Part model, mm, in its own coordinate system. Give positions to 0.01 mm unless a question says otherwise; leave off trailing zeros. Write each loop counter-clockwise with the first axis right and the second up, starting at its lowest first coordinate (ties: lowest second). Pieces come first, ordered by that corner, then holes. Notation, with made-up numbers: M -19,-13 L 21,-13 A16 ccw 21,15 Z; hole C 38.5,-29 d1. An arc over 180 degrees is marked long. Answer as CSV lines item,"result". Start each with the question number.
1) Slice it at B-B, the plane y = 65. Give the cut face in (x, z).
2) Slice it at D-D, the plane y = -54. Give the cut face in (x, z).
3) Wall check: line 1 along Y through (x, z) = (0, 1.3); line 2 along X through (y, z) = (-13, 22); line 3 along Y through (x, z) = (-40.5, 14.5). Give the ranges that are in metal, low to high. Write a range as from..to.
4) Pin check, flat tips, straight feed: pin 1 Ø1.5 at (x, y) = (9.5, -29.5) entering from -Z; pin 2 Ø10 at (y, z) = (41.5, 10.5) entering from -X; pin 3 Ø1.6 at (y, z) = (68, 1.5) entering from +X; pin 4 Ø1.6 at (y, z) = (63.5, 1.5) entering from -X. Stop position of each tip, or through.
5) Slice it at A-A, the plane x = 0. Give the cut face in (y, z).
6) Slice it at C-C, the plane z = 19.5. Give the cut face in (x, y).
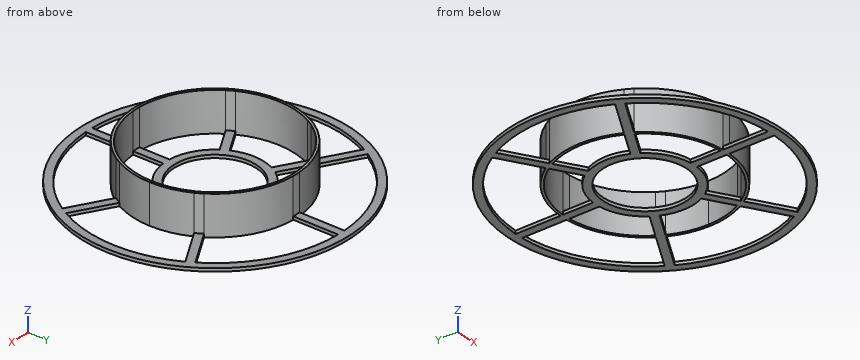
```python
from build123d import *

# Parameters (mm, degrees)
F0_R     = 85
F0_R_2   = 26
F1_DEPTH = 2
F2_DEPTH = 25


with BuildPart() as f1:
    # F0 (on Top) → F1 (new body)
    with BuildSketch(Plane.XY):
        Circle(F0_R)
        with BuildLine():
            ThreePointArc((43.384432, 27.934765), (44.686911, 25.8), (45.884432, 23.604638))
            Line((45.884432, 23.604638), (70.498195, 37.8154))
            ThreePointArc((70.498195, 37.8154), (80, 0), (70.498195, -37.8154))
            Line((70.498195, -37.8154), (45.884432, -23.604638))
            ThreePointArc((45.884432, -23.604638), (44.686911, -25.8), (43.384432, -27.934765))
            Line((43.384432, -27.934765), (67.998195, -42.145527))
            ThreePointArc((67.998195, -42.145527), (40, -69.282032), (2.5, -79.960928))
            Line((2.5, -79.960928), (2.5, -51.539402))
            ThreePointArc((2.5, -51.539402), (0, -51.6), (-2.5, -51.539402))
            Line((-2.5, -51.539402), (-2.5, -79.960928))
            ThreePointArc((-2.5, -79.960928), (-40, -69.282032), (-67.998195, -42.145527))
            Line((-67.998195, -42.145527), (-43.384432, -27.934765))
            ThreePointArc((-43.384432, -27.934765), (-44.686911, -25.8), (-45.884432, -23.604638))
            Line((-45.884432, -23.604638), (-70.498195, -37.8154))
            ThreePointArc((-70.498195, -37.8154), (-80, 0), (-70.498195, 37.8154))
            Line((-70.498195, 37.8154), (-45.884432, 23.604638))
            ThreePointArc((-45.884432, 23.604638), (-44.686911, 25.8), (-43.384432, 27.934765))
            Line((-43.384432, 27.934765), (-67.998195, 42.145527))
            ThreePointArc((-67.998195, 42.145527), (-40, 69.282032), (-2.5, 79.960928))
            Line((-2.5, 79.960928), (-2.5, 51.539402))
            ThreePointArc((-2.5, 51.539402), (0, 51.6), (2.5, 51.539402))
            Line((2.5, 51.539402), (2.5, 79.960928))
            ThreePointArc((2.5, 79.960928), (40, 69.282032), (67.998195, 42.145527))
            Line((67.998195, 42.145527), (43.384432, 27.934765))
        make_face(mode=Mode.SUBTRACT)
        with BuildLine():
            Line((28.009344, 13.284451), (44.49711, 22.803667))
            ThreePointArc((44.49711, 22.803667), (43.30127, 25), (41.99711, 27.133794))
            Line((41.99711, 27.133794), (25.509344, 17.614578))
            ThreePointArc((25.509344, 17.614578), (15.5, 26.846788), (2.5, 30.899029))
            Line((2.5, 30.899029), (2.5, 49.937461))
            ThreePointArc((2.5, 49.937461), (0, 50), (-2.5, 49.937461))
            Line((-2.5, 49.937461), (-2.5, 30.899029))
            ThreePointArc((-2.5, 30.899029), (-15.5, 26.846788), (-25.509344, 17.614578))
            Line((-25.509344, 17.614578), (-41.99711, 27.133794))
            ThreePointArc((-41.99711, 27.133794), (-43.30127, 25), (-44.49711, 22.803667))
            Line((-44.49711, 22.803667), (-28.009344, 13.284451))
            ThreePointArc((-28.009344, 13.284451), (-31, 0), (-28.009344, -13.284451))
            Line((-28.009344, -13.284451), (-44.49711, -22.803667))
            ThreePointArc((-44.49711, -22.803667), (-43.30127, -25), (-41.99711, -27.133794))
            Line((-41.99711, -27.133794), (-25.509344, -17.614578))
            ThreePointArc((-25.509344, -17.614578), (-15.5, -26.846788), (-2.5, -30.899029))
            Line((-2.5, -30.899029), (-2.5, -49.937461))
            ThreePointArc((-2.5, -49.937461), (0, -50), (2.5, -49.937461))
            Line((2.5, -49.937461), (2.5, -30.899029))
            ThreePointArc((2.5, -30.899029), (15.5, -26.846788), (25.509344, -17.614578))
            Line((25.509344, -17.614578), (41.99711, -27.133794))
            ThreePointArc((41.99711, -27.133794), (43.30127, -25), (44.49711, -22.803667))
            Line((44.49711, -22.803667), (28.009344, -13.284451))
            ThreePointArc((28.009344, -13.284451), (31, 0), (28.009344, 13.284451))
        make_face()
        Circle(F0_R_2, mode=Mode.SUBTRACT)
    extrude(amount=F1_DEPTH)

    # F0 (on Top) → F2 (join)
    with BuildSketch(Plane.XY):
        with BuildLine():
            ThreePointArc((45.884432, -23.604638), (50.150756, -12.143379), (51.6, 0))
            ThreePointArc((51.6, 0), (50.150756, 12.143379), (45.884432, 23.604638))
            ThreePointArc((45.884432, 23.604638), (44.686911, 25.8), (43.384432, 27.934765))
            ThreePointArc((43.384432, 27.934765), (25.8, 44.686911), (2.5, 51.539402))
            ThreePointArc((2.5, 51.539402), (0, 51.6), (-2.5, 51.539402))
            ThreePointArc((-2.5, 51.539402), (-25.8, 44.686911), (-43.384432, 27.934765))
            ThreePointArc((-43.384432, 27.934765), (-44.686911, 25.8), (-45.884432, 23.604638))
            ThreePointArc((-45.884432, 23.604638), (-51.6, 0), (-45.884432, -23.604638))
            ThreePointArc((-45.884432, -23.604638), (-44.686911, -25.8), (-43.384432, -27.934765))
            ThreePointArc((-43.384432, -27.934765), (-25.8, -44.686911), (-2.5, -51.539402))
            ThreePointArc((-2.5, -51.539402), (0, -51.6), (2.5, -51.539402))
            ThreePointArc((2.5, -51.539402), (25.8, -44.686911), (43.384432, -27.934765))
            ThreePointArc((43.384432, -27.934765), (44.686911, -25.8), (45.884432, -23.604638))
        make_face()
        with BuildLine():
            ThreePointArc((44.49711, 22.803667), (48.604812, 11.72912), (50, 0))
            ThreePointArc((50, 0), (48.604812, -11.72912), (44.49711, -22.803667))
            ThreePointArc((44.49711, -22.803667), (43.30127, -25), (41.99711, -27.133794))
            ThreePointArc((41.99711, -27.133794), (25, -43.30127), (2.5, -49.937461))
            ThreePointArc((2.5, -49.937461), (0, -50), (-2.5, -49.937461))
            ThreePointArc((-2.5, -49.937461), (-25, -43.30127), (-41.99711, -27.133794))
            ThreePointArc((-41.99711, -27.133794), (-43.30127, -25), (-44.49711, -22.803667))
            ThreePointArc((-44.49711, -22.803667), (-50, 0), (-44.49711, 22.803667))
            ThreePointArc((-44.49711, 22.803667), (-43.30127, 25), (-41.99711, 27.133794))
            ThreePointArc((-41.99711, 27.133794), (-25, 43.30127), (-2.5, 49.937461))
            ThreePointArc((-2.5, 49.937461), (0, 50), (2.5, 49.937461))
            ThreePointArc((2.5, 49.937461), (25, 43.30127), (41.99711, 27.133794))
            ThreePointArc((41.99711, 27.133794), (43.30127, 25), (44.49711, 22.803667))
        make_face(mode=Mode.SUBTRACT)
    extrude(amount=F2_DEPTH)


solid = f1.part
```
Found:
1,outline,"M -54.77,0 L -46.64,0 L -46.64,2 L -54.77,2 Z; M -2.5,0 L 2.5,0 L 2.5,2 L -2.5,2 Z; M 46.64,0 L 54.77,0 L 54.77,2 L 46.64,2 Z"
2,outline,"M -65.64,0 L -59.03,0 L -59.03,2 L -65.64,2 Z; M -2.5,0 L 2.5,0 L 2.5,2 L -2.5,2 Z; M 59.03,0 L 65.64,0 L 65.64,2 L 59.03,2 Z"
3,line 1,"-85..-26, 26..85"
3,line 2,"-49.94..-48.28, 48.28..49.94"
3,line 3,"-31.97..-29.32, 29.32..31.97"
4,pin 1,"z = 0"
4,pin 2,"x = -36.47"
4,pin 3,"x = 52.05"
4,pin 4,"x = -57.39"
5,outline,"M -85,0 L -26,0 L -26,2 L -50,2 L -50,25 L -51.6,25 L -51.6,2 L -85,2 Z; M 26,0 L 85,0 L 85,2 L 51.6,2 L 51.6,25 L 50,25 L 50,2 L 26,2 Z"
6,outline,"M -45.88,-23.6 A51.6 ccw -43.38,-27.93 A51.6 ccw -2.5,-51.54 A51.6 ccw 2.5,-51.54 A51.6 ccw 43.38,-27.93 A51.6 ccw 45.88,-23.6 A51.6 ccw 51.6,0 A51.6 ccw 45.88,23.6 A51.6 ccw 43.38,27.93 A51.6 ccw 2.5,51.54 A51.6 ccw -2.5,51.54 A51.6 ccw -43.38,27.93 A51.6 ccw -45.88,23.6 A51.6 ccw Z; hole M -44.5,-22.8 A50 ccw -42,-27.13 A50 ccw -2.5,-49.94 A50 ccw 2.5,-49.94 A50 ccw 42,-27.13 A50 ccw 44.5,-22.8 A50 ccw 44.5,22.8 A50 ccw 42,27.13 A50 ccw 2.5,49.94 A50 ccw -2.5,49.94 A50 ccw -42,27.13 A50 ccw -44.5,22.8 A50 ccw Z"
